Verification items for the finished model (mm, model axes). A direction names the side the tool comes from. Coordinates: 2 decimals unless noted, no trailing zeros. Order: outer loops, then holes, each group sorted by start corner. A loop starts at its lowest first (then second) coordinate and runs counter-clockwise, first axis right, second up. Notation, with made-up numbers: M 56,17 L 81,17 A32 cw 81,54 Z; hole C -8.5,37.5 d4. An arc over 180 degrees is marked long. Use one line per item in the form item = value. Start each with the question number.
Autodesk Inventor part; units mm, degrees
ref_plane "Work Plane1" through (-24.9, -24.9, 7.7) normal (0, 0, 1) x (1, 0, 0)
ref_plane "YZ Plane" through (0, 0, 0) normal (1, 0, 0) x (0, 1, 0)
ref_plane "XZ Plane" through (0, 0, 0) normal (0, 1, 0) x (-1, 0, 0)
sketch "Sketch1" plane through (0, 0, 0) normal (0, 0, 1) x (1, 0, 0)
  circle A0 centre (-10, 20.9) radius 1.875
  circle A1 centre (-10, -20.9) radius 1.875
  circle A2 centre (10, 20.9) radius 1.875
  circle A3 centre (10, -20.9) radius 1.875
  circle A4 centre (20.8, -14.4) radius 2.075
  circle A5 centre (20.8, 14.4) radius 2.075
  circle A6 centre (-20.8, 14.4) radius 2.075
  circle A7 centre (-20.8, -14.4) radius 2.075
  line L0 (16.9, -16.9) -> (-16.9, -16.9)
  line L1 (-16.9, -16.9) -> (-16.9, 16.9)
  line L2 (-16.9, 16.9) -> (16.9, 16.9)
  line L3 (16.9, 16.9) -> (16.9, -16.9)
  line L4 (-17.05, 24.9) -> (-17.05, 22.55)
  line L5 (-17.05, 22.55) -> (-22.55, 17.05)
  line L6 (-22.55, 17.05) -> (-24.9, 17.05)
  line L7 (-24.9, 17.05) -> (-24.9, -17.05)
  line L8 (-24.9, -17.05) -> (-22.55, -17.05)
  line L9 (-22.55, -17.05) -> (-17.05, -22.55)
  line L10 (-17.05, -22.55) -> (-17.05, -24.9)
  line L11 (-17.05, -24.9) -> (17.05, -24.9)
  line L12 (17.05, -24.9) -> (17.05, -22.55)
  line L13 (17.05, -22.55) -> (22.55, -17.05)
  line L14 (22.55, -17.05) -> (24.9, -17.05)
  line L15 (24.9, -17.05) -> (24.9, 17.05)
  line L16 (24.9, 17.05) -> (22.55, 17.05)
  line L17 (22.55, 17.05) -> (17.05, 22.55)
  line L18 (17.05, 22.55) -> (17.05, 24.9)
  line L19 (17.05, 24.9) -> (-17.05, 24.9)
  line L20 (24.825, 16.975) -> (24.825, -16.975)
  line L21 (24.825, -16.975) -> (22.5189, -16.975)
  line L22 (22.5189, -16.975) -> (16.975, -22.5189)
  line L23 (16.975, -22.5189) -> (16.975, -24.825)
  line L24 (16.975, -24.825) -> (-16.975, -24.825)
  line L25 (-16.975, -24.825) -> (-16.975, -22.5189)
  line L26 (-16.975, -22.5189) -> (-22.5189, -16.975)
  line L27 (-22.5189, -16.975) -> (-24.825, -16.975)
  line L28 (-24.825, -16.975) -> (-24.825, 16.975)
  line L29 (-24.825, 16.975) -> (-22.5189, 16.975)
  line L30 (-22.5189, 16.975) -> (-16.975, 22.5189)
  line L31 (-16.975, 22.5189) -> (-16.975, 24.825)
  line L32 (-16.975, 24.825) -> (16.975, 24.825)
  line L33 (16.975, 24.825) -> (16.975, 22.5189)
  line L34 (16.975, 22.5189) -> (22.5189, 16.975)
  line L35 (22.5189, 16.975) -> (24.825, 16.975)
  line L36 (22.5189, -16.975) -> (22.5189, 16.975)
  line L37 (16.975, 22.5189) -> (-16.975, 22.5189)
  line L38 (-22.5189, 16.975) -> (-22.5189, -16.975)
  line L39 (-16.975, -22.5189) -> (16.975, -22.5189)
  line L40 (16.975, 24.825) -> (24.825, 24.825)
  line L41 (24.825, 24.825) -> (24.825, 16.975)
  line L42 (24.825, 24.825) -> (14.825, 24.825)
  line L43 (14.825, 24.825) -> (14.825, 21.575)
  line L44 (21.575, 14.825) -> (24.825, 14.825)
  line L45 (24.825, 14.825) -> (24.825, 24.825)
  line L46 (14.825, 21.575) -> (21.575, 14.825)
  line L47 (-21.575, 14.825) -> (-14.825, 21.575)
  line L48 (-14.825, 21.575) -> (-14.825, 24.825)
  line L49 (-24.825, 14.825) -> (-21.575, 14.825)
  line L50 (-14.825, -21.575) -> (-21.575, -14.825)
  line L51 (-21.575, -14.825) -> (-24.825, -14.825)
  line L52 (-14.825, -24.825) -> (-14.825, -21.575)
  line L53 (21.575, -14.825) -> (14.825, -21.575)
  line L54 (14.825, -21.575) -> (14.825, -24.825)
  line L55 (24.825, -14.825) -> (21.575, -14.825)
  point P0 (0, 0)
  point P1 (14.825, 14.825)
  point P2 (22.5189, 14.825)
  point P3 (22.5189, -14.825)
  point P4 (14.825, -22.5189)
  point P5 (-14.825, -22.5189)
  point P6 (-22.5189, -14.825)
  point P7 (-22.5189, 14.825)
  point P8 (-14.825, 22.5189)
  point P9 (14.825, 22.5189)
  dimension "d0" = 0.075
  dimension "d3" = 360
  dimension "d5" = 10
  dimension "d6" = 10
  dimension "d7" = 6.75
  dimension "d8" = 6.75
  dimension "d11" = 360
ref_plane "Work Plane1" through (-24.9, -24.9, 7.7) normal (0, 0, 1) x (1, 0, 0)
extrude "Extrusion1" add sketch "Sketch1" along normal blind 34.325 from surface at 7.7 contours L37 A0 | A0 L37 L48 L32 L43 A2 | A2 L37 | L48 L47 A6 L38 L30 L37 | L37 L31 L32 L48 | L43 L32 L33 L37 | L37 L34 L36 A5 L46 L43 | L38 A6 L49 L28 L29 | L47 L49 L38 A6 | L38 L49 A6 | L35 L20 L44 A5 L36 | A5 L36 L44 L46 | L49 A6 L38 A7 L51 L28 | L49 L38 A6 | A5 L44 L36 | L36 L44 A5 | A5 L44 L20 L55 A4 L36 | L51 A7 L38 L27 L28 | L38 L51 A7 | A4 L55 L36 | L51 L38 A7 | L51 L50 A7 L38 | L20 L21 L36 A4 L55 | L53 L55 L36 A4 | A4 L36 L22 L39 L54 L53 | L55 A4 L36 | L38 A7 L50 L52 L39 L26 | L39 L52 L24 L25 | L54 L24 L52 L39 A1 A3 | L39 L23 L24 L54 | A3 L39 | L39 A1 picked at (-9.805, 22.5731) picked at (9.805, 22.5731) picked at (-20.715, 15.8728) picked at (20.715, 15.8728) picked at (-20.715, -15.8728) picked at (20.715, -15.8728) picked at (10.195, -22.5731) picked at (-9.805, -22.5731)
properties part number "Tunnel Vertical"
1. Depth check by flat-ended pin: P1, Ø1.8, axis at y = -23.5, z = 31.5, coming from the +X side (3 decimals); P2, Ø1.8, axis at x = -24, z = 22, coming from the +Y side (3 decimals); P3, Ø1, axis at x = 22, z = 32, coming from the -Y side. Enter the tip coordinate at first touch or a pass-through.
2. Cross-section at A-A on y = 3. Enter the section's corners in (x, z) (3 decimals).
3. Tool access check on faces 1 (the flat face through (-22.519, 0, 25)), 2 (the flat face through (-24, 16.975, 25)), 3 (the flat face through (24, -16.975, 25)), 4 (the flat face through (24, 16.975, 25)), 5 (the flat face through (-24, -16.975, 25)). Record the directions out of +Z, -Z, +X, -X, +Y, -Y that give a thin tool (end or side, any length) a straight path to the whole face; none if there is none.
4. Material ranges on line 1 along Y through (x, z) = (6, 29) (3 decimals); line 2 along Y through (x, z) = (-18, 13.5), recorded low to high.
Final values:
q1.P1 = 16.975
q1.P2 = 16.975
q1.P3 = -17.99
q2.outline = M -24.825,7.7 L -22.519,7.7 L -22.519,42.025 L -24.825,42.025 Z; M 22.519,7.7 L 24.825,7.7 L 24.825,42.025 L 22.519,42.025 Z
q3.face_1 = +Z, -Z
q3.face_2 = +Z, -Z, -X, +Y
q3.face_3 = +Z, -Z, +X, -Y
q3.face_4 = +Z, -Z, +X, +Y
q3.face_5 = +Z, -Z, -X, -Y
q4.line_1 = -24.825 to -22.519, 22.519 to 24.825
q4.line_2 = -21.49 to -18.4, 18.4 to 21.49
